Read the model definition and answer for the solid it produces. Units are mm, in the model's axes. Coordinates: 2 decimals unless noted, no trailing zeros. Write each loop counter-clockwise with the first axis right and the second up, starting at its lowest first coordinate (ties: lowest second). Pieces come first, ordered by that corner, then holes.
(1) The part is cut by section A-A, the plane y = -13. Determine the outline of the cut face in (x, z).
(2) Determine the mould class of faces 1 (the flat face through (-16, 0, 1)), 2 (the flat face through (16, 0, 1)), 3 (the cylindrical face through (13.222, -6.925, 0.784)) for opening direction X: pulls with the +X half, pulls with the -X half, needs draft (parallel to the pull), parting line crosses it, or undercut.
(3) Straight lines are drawn through the part: line 1 along Y through (x, z) = (5.8, 1); line 2 along X through (y, z) = (-1.5, 1.55); line 3 along Y through (x, z) = (11, 1.55). For each, find the intervals that lie inside material, in ascending order.
(4) The part is cut by section D-D, the plane z = 1.35. State how many separate pieces and enclosed holes the cut face has, and give its area (3 significant figures).
(5) The part is cut by section C-C, the plane y = 15.18. Determine the outline of the cut face in (x, z), and give its area (3 significant figures).
(6) The part is cut by section B-B, the plane x = -10.2. Determine the outline of the cut face in (y, z), and give its area (3 significant figures).
```python
from build123d import *

# Parameters (mm, degrees)
SKETCH_3_W      = 32
SKETCH_3_H      = 32
SKETCH_3_R      = 1.5
SKETCH_3_R_2    = 0.68
SKETCH_3_R_3    = 0.5
EXTRUDE_5_DEPTH = 1.59


with BuildPart() as part:
    # 草图3 → 凸台-拉伸5 (new body)
    with BuildSketch(Plane.XY):
        Rectangle(SKETCH_3_W, SKETCH_3_H)
        with Locations((-10.2, 13)):
            Circle(SKETCH_3_R, mode=Mode.SUBTRACT)
        with Locations((10.2, 13)):
            Circle(SKETCH_3_R, mode=Mode.SUBTRACT)
        with Locations((10.2, -13)):
            Circle(SKETCH_3_R, mode=Mode.SUBTRACT)
        with Locations((-10.2, -13)):
            Circle(SKETCH_3_R, mode=Mode.SUBTRACT)
        with Locations((-12.594133286, 9.217216134)):
            Circle(SKETCH_3_R_2, mode=Mode.SUBTRACT)
        with Locations((-12.594133286, 6.664068101)):
            Circle(SKETCH_3_R_2, mode=Mode.SUBTRACT)
        with Locations((-12.594133286, 4.110920068)):
            Circle(SKETCH_3_R_2, mode=Mode.SUBTRACT)
        with Locations((-12.594133286, 1.492306701)):
            Circle(SKETCH_3_R_2, mode=Mode.SUBTRACT)
        with Locations((-12.594133286, -1.492306701)):
            Circle(SKETCH_3_R_2, mode=Mode.SUBTRACT)
        with Locations((-12.594133286, -4.110920068)):
            Circle(SKETCH_3_R_2, mode=Mode.SUBTRACT)
        with Locations((-12.594133286, -6.664068101)):
            Circle(SKETCH_3_R_2, mode=Mode.SUBTRACT)
        with Locations((-12.594133286, -9.217216134)):
            Circle(SKETCH_3_R_2, mode=Mode.SUBTRACT)
        with Locations((12.594133286, -9.217216134)):
            Circle(SKETCH_3_R_2, mode=Mode.SUBTRACT)
        with Locations((12.594133286, -6.664068101)):
            Circle(SKETCH_3_R_2, mode=Mode.SUBTRACT)
        with Locations((12.594133286, -4.110920068)):
            Circle(SKETCH_3_R_2, mode=Mode.SUBTRACT)
        with Locations((12.594133286, -1.492306701)):
            Circle(SKETCH_3_R_2, mode=Mode.SUBTRACT)
        with Locations((12.594133286, 1.492306701)):
            Circle(SKETCH_3_R_2, mode=Mode.SUBTRACT)
        with Locations((12.594133286, 4.110920068)):
            Circle(SKETCH_3_R_2, mode=Mode.SUBTRACT)
        with Locations((12.594133286, 6.664068101)):
            Circle(SKETCH_3_R_2, mode=Mode.SUBTRACT)
        with Locations((12.594133286, 9.217216134)):
            Circle(SKETCH_3_R_2, mode=Mode.SUBTRACT)
        with Locations((-5.8, 15.18)):
            Circle(SKETCH_3_R_3, mode=Mode.SUBTRACT)
        with Locations((0, 15.18)):
            Circle(SKETCH_3_R_3, mode=Mode.SUBTRACT)
        with Locations((-3.193886251, 15.18)):
            Circle(SKETCH_3_R_3, mode=Mode.SUBTRACT)
        with Locations((3.193886251, 15.18)):
            Circle(SKETCH_3_R_3, mode=Mode.SUBTRACT)
        with Locations((5.8, 15.18)):
            Circle(SKETCH_3_R_3, mode=Mode.SUBTRACT)
        with Locations((5.8, -15.18)):
            Circle(SKETCH_3_R_3, mode=Mode.SUBTRACT)
        with Locations((3.193886251, -15.18)):
            Circle(SKETCH_3_R_3, mode=Mode.SUBTRACT)
        with Locations((0, -15.18)):
            Circle(SKETCH_3_R_3, mode=Mode.SUBTRACT)
        with Locations((-3.193886251, -15.18)):
            Circle(SKETCH_3_R_3, mode=Mode.SUBTRACT)
        with Locations((-5.8, -15.18)):
            Circle(SKETCH_3_R_3, mode=Mode.SUBTRACT)
    extrude(amount=EXTRUDE_5_DEPTH)


solid = part.part
```
Computed:
1. outline: (-16, 0) - (-11.7, 0) - (-11.7, 1.59) - (-16, 1.59) - close; (-8.7, 0) - (8.7, 0) - (8.7, 1.59) - (-8.7, 1.59) - close; (11.7, 0) - (16, 0) - (16, 1.59) - (11.7, 1.59) - close
2. face 1: pulls with the -X half
2. face 2: pulls with the +X half
2. face 3: undercut
3. line 1: y = -16 to -15.68, -14.68 to 14.68, 15.68 to 16
3. line 2: x = -16 to -13.27, -11.91 to 11.91, 13.27 to 16
3. line 3: y = -16 to -14.27, -11.73 to 11.73, 14.27 to 16
4. separate pieces: 1
4. enclosed holes: 30
4. area: 965 mm2
5. outline: (-16, 0) - (-6.3, 0) - (-6.3, 1.59) - (-16, 1.59) - close; (-5.3, 0) - (-3.69, 0) - (-3.69, 1.59) - (-5.3, 1.59) - close; (-2.69, 0) - (-0.5, 0) - (-0.5, 1.59) - (-2.69, 1.59) - close; (0.5, 0) - (2.69, 0) - (2.69, 1.59) - (0.5, 1.59) - close; (3.69, 0) - (5.3, 0) - (5.3, 1.59) - (3.69, 1.59) - close; (6.3, 0) - (16, 0) - (16, 1.59) - (6.3, 1.59) - close
5. area: 42.9 mm2
6. outline: (-16, 0) - (-14.5, 0) - (-14.5, 1.59) - (-16, 1.59) - close; (-11.5, 0) - (11.5, 0) - (11.5, 1.59) - (-11.5, 1.59) - close; (14.5, 0) - (16, 0) - (16, 1.59) - (14.5, 1.59) - close
6. area: 41.3 mm2
